Geometry: see drawing. Coordinates: mm, zero at the bounding-box minimum. Give positions to 0.01 mm unless a question says otherwise; leave off trailing zeros. Write each loop counter-clockwise with the first axis right and the second up, starting at its lowest first coordinate (ties: lowest second). Pieces come first, ordered by that corner, then holes. Notation, with made-up numbers: (8, 56.5) -> (39, 56.5) arc R25 cw to (39, 89.5) -> close; hole circle Ø2 at (28, 67.25). An arc over 180 degrees is marked (long way). Answer as a JSON object with one key per item and string values. Group by question number.
Item 1: Section query A-A on x = 40. Return the cut outline in (y, z), plus the area to 3 significant figures.
Item 2: First-contact query: pin 1 Ø0.5 at (x, z) = (18, 0.5) entering from -Y; pin 2 Ø0.5 at (y, z) = (14.5, 0.5) entering from +X. Flat tips, straight axial feed; report the tip coordinate or a pass-through.
Item 3: Section query B-B on y = 23.5. Return the cut outline in (x, z), plus the area to 3 significant figures.
Item 4: Ray query, probe 1 along Y at (x, z) = (41.5, 0.9); probe 2 along X at (y, z) = (13.5, 0.65). Return the intervals inside material, ascending. Write a range as from..to.
Item 5: Section query C-C on z = 0.4. Return the cut outline in (x, y).
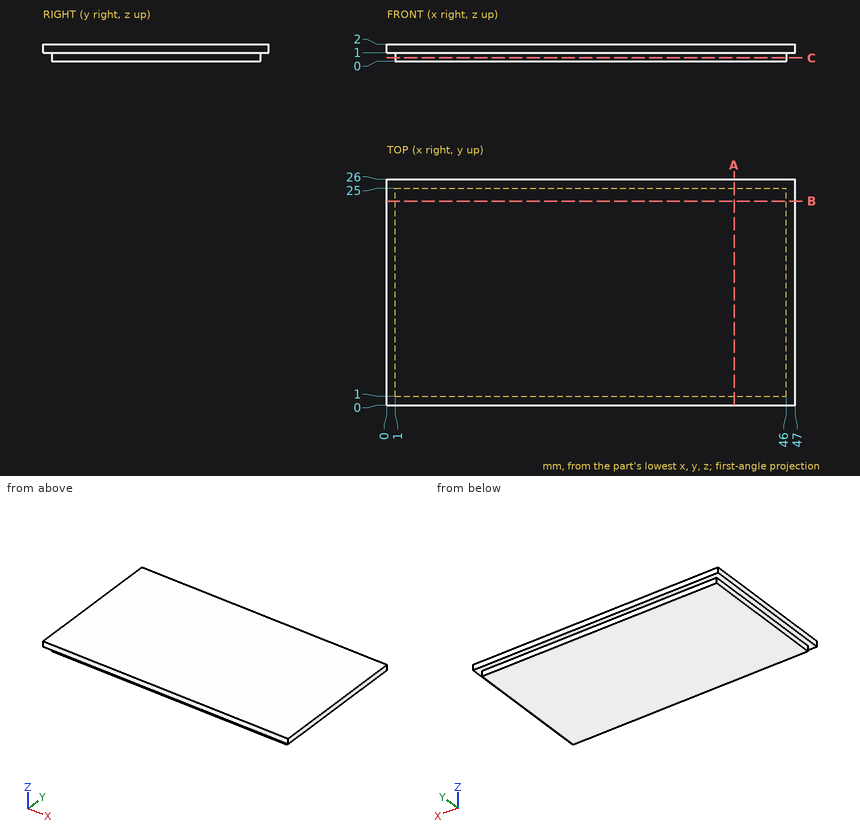
Worked answers:
{
 "1": {"outline": "(0, 1) -> (1, 1) -> (1, 0) -> (25, 0) -> (25, 1) -> (26, 1) -> (26, 2) -> (0, 2) -> close", "area": "50.0 mm^2"},
 "2": {"pin 1": "y = 1", "pin 2": "x = 46"},
 "3": {"outline": "(0, 1) -> (1, 1) -> (1, 0) -> (46, 0) -> (46, 1) -> (47, 1) -> (47, 2) -> (0, 2) -> close", "area": "92.0 mm^2"},
 "4": {"probe 1": "1..25", "probe 2": "1..46"},
 "5": {"outline": "(1, 1) -> (46, 1) -> (46, 25) -> (1, 25) -> close"}
}
